Geometry: final body of the model. Coordinates: model frame, mm. Face numbers are marked on the shaded views. Give positions to 0.01 mm unless a question says otherwise; leave off trailing zeros. Loops run counter-clockwise (first coordinate to the right, second up) from the corner with the lowest first, then second, coordinate; pieces in that order, holes last.
from build123d import *

# Parameters (mm, degrees)
F0_R     = 25
F0_R_2   = 15
F1_DEPTH = 100
F2_R     = 25
F2_R_2   = 15
F3_R     = 45
F3_R_2   = 25
F4_DEPTH = 50
F5_R     = 5
F6_R     = 5


with BuildPart() as f1:
    # F0 (on Right) → F1 (new body)
    with BuildSketch(Plane.YZ):
        with Locations((0, 39.787832)):
            Circle(F0_R)
        with Locations((0, 39.787832)):
            Circle(F0_R_2, mode=Mode.SUBTRACT)
    extrude(amount=F1_DEPTH)

    # F2 (on face) + F3 (on face) → F4 (join)
    with BuildSketch(Plane.YZ.offset(100)):
        with Locations((0, 39.787832)):
            Circle(F2_R)
        with Locations((0, 39.787832)):
            Circle(F2_R_2, mode=Mode.SUBTRACT)
    with BuildSketch(Plane.YZ.offset(100)):
        with Locations((0, 39.787832)):
            Circle(F3_R)
        with Locations((0, 39.787832)):
            Circle(F3_R_2, mode=Mode.SUBTRACT)
    extrude(amount=F4_DEPTH)

    # F5
    f5_edges = [f1.edges().sort_by_distance(p)[0] for p in [
        (100, -45, 39.787832),
        (0, -25, 39.787832),
    ]]
    fillet(f5_edges, radius=F5_R)

    # F6
    f6_edges = [f1.edges().sort_by_distance(p)[0] for p in [
        (150, -45, 39.787832),
    ]]
    fillet(f6_edges, radius=F6_R)


solid = f1.part
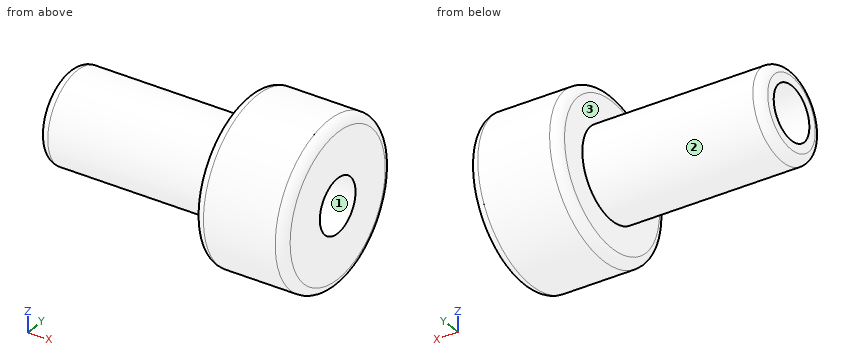
Item 1: Ray query, probe 1 along Z at (x, y) = (57, 0); probe 2 along Z at (x, y) = (112, 0); probe 3 along X at (y, z) = (1, 72). Return the intervals inside material, ascending.
Values follow:
probe 1: z = 14.79 to 24.79, 54.79 to 64.79
probe 2: z = -5.21 to 24.79, 54.79 to 84.79
probe 3: x = 100 to 150
Item 2: Draft query along Z for the marked faces 1, 2 and 3. Return one class per face: +Z half, -Z half, draft (parallel to the pull), parting line (faces both ways), or undercut.
Values follow:
face 1: undercut
face 2: parting line
face 3: draft
Item 3: Pin query (flat end, axial travel): pin 1 (1 mm diameter, centred on x = 36.5, y = -20, fed in from -Z); pin 2 (5 mm diameter, centred on x = 118.5, y = -0.5, fed in from +Z); pin 3 (12 mm diameter, centred on x = 101, y = -33, fed in from +Z). Return the tip coordinate at first contact, or that it passes through.
Values follow:
pin 1: stops at z = 24.14
pin 2: stops at z = 84.79
pin 3: stops at z = 75.08
Item 4: Section query B-B on x = 14. Return loops of the section in (y, z).
Values follow:
outline: circle Ø50 at (0, 39.79); hole circle Ø30 at (0, 39.79)
Item 5: Section query C-C on x = 111.5. Return loops of the section in (y, z), plus the area to 3 significant figures.
Values follow:
outline: circle Ø90 at (0, 39.79); hole circle Ø30 at (0, 39.79)
area: 5,650 mm2
Item 6: Section query A-A on y = 0. Return loops of the section in (x, z).
Values follow:
outline: (0, 19.79) arc R5 ccw to (5, 14.79) - (100, 14.79) - (100, -0.21) arc R5 ccw to (105, -5.21) - (145, -5.21) arc R5 ccw to (150, -0.21) - (150, 24.79) - (0, 24.79) - close; (0, 54.79) - (150, 54.79) - (150, 79.79) arc R5 ccw to (145, 84.79) - (105, 84.79) arc R5 ccw to (100, 79.79) - (100, 64.79) - (5, 64.79) arc R5 ccw to (0, 59.79) - close
